CAD build for the part. Positions are in the model's coordinates, mm. A direction names the side the tool comes from. Round coordinates to 2 decimals unless told otherwise and drop trailing zeros. Loops run counter-clockwise (first coordinate to the right, second up) from the corner with the lowest first, then second, coordinate; pieces in that order, holes last.
```python
from build123d import *

# Parameters (mm, degrees)
F0_W     = 310.82517
F0_H     = 231.34768
F1_DEPTH = 189
F2_R     = 20
F3_R     = 13.644912
F3_R_2   = 26.127936
F3_R_3   = 16.173919
F4_DEPTH = 189.001
F5_T     = -10
F6_R     = 32.715141
F7_DEPTH = 189.001


with BuildPart() as f1:
    # F0 (on Front) → F1 (new body)
    with BuildSketch(Plane.XZ):
        Rectangle(F0_W, F0_H)
    extrude(amount=F1_DEPTH)

    # F2
    f2_edges = [f1.edges().sort_by_distance(p)[0] for p in [
        (155.412585, -94.5, 115.67384),
        (-155.412585, -94.5, 115.67384),
        (0, 0, 115.67384),
        (0, -189, 115.67384),
    ]]
    fillet(f2_edges, radius=F2_R)

    # F3 (on face) → F4 (cut, through all)
    with BuildSketch(Plane.XZ.offset(189)):
        with Locations((-105.628975, -68.58331)):
            Circle(F3_R)
        with Locations((-9.658518, -9.867162)):
            Circle(F3_R_2)
        with Locations((92.311822, 54.978933)):
            Circle(F3_R_3)
    extrude(amount=-F4_DEPTH, mode=Mode.SUBTRACT)

    # F5
    f5_openings = [f1.faces().sort_by_distance(p)[0] for p in [
        (0, -94.5, -115.67384),
    ]]
    offset(amount=F5_T, openings=f5_openings)

    # F6 (on face) → F7 (cut, through all)
    with BuildSketch(Plane(origin=(0, 0, 0), x_dir=(-1, 0, 0), z_dir=(0, 1, 0))):
        with Locations((-73.95748, -58.360144)):
            Circle(F6_R)
    extrude(amount=-F7_DEPTH, mode=Mode.SUBTRACT)


solid = f1.part
```
Item 1: 3-axis set-ups, long thin cutter, end or side, ignore diameter. For faces 4 (the cylindrical face through (2.036, -175.993, 102.822)), 5 (the cylindrical face through (-149.71, -95.82, 109.66)), 6 (the cylindrical face through (142.56, -95.68, 102.67)): which of +Z, -Z, +X, -X, +Y, -Y reach the whole face in a straight line?
Answers follow:
face 4: none
face 5: +Z, -X, +Y, -Y
face 6: -Z
Item 2: Flat gauge pins, fed straight in: P1, Ø1.5, axis at x = 123, y = -47.5, coming from the -Z side; P2, Ø19.5, axis at x = 92.31, z = 54.98, coming from the -Y side; P3, Ø1, axis at x = -20.5, y = -82, coming from the -Z side. Where does each tip first touch, or does it go through?
Answers follow:
P1: stops at z = 105.67
P2: passes through
P3: stops at z = -44.48
Item 3: Probe line 1 (X direction, y = -63, z = -105); line 2 (Y direction, x = -39, z = 16); line 3 (X direction, y = -127, z = 57). List the from-to ranges inside material, lowest first.
Answers follow:
line 1: x = -155.41 to -145.41, 145.41 to 155.41
line 2: y = -189 to -179, -10 to 0
line 3: x = -155.41 to -145.41, 66.22 to 76.26, 108.36 to 118.41, 145.41 to 155.41
Item 4: Cut at B-B, the plane x = 70. Give the cut face in (y, z).
Answers follow:
outline: (-189, -115.67) - (-179, -115.67) - (-179, -90.84) - (-189, -90.84) - close; (-189, -25.89) - (-179, -25.89) - (-179, 41.29) - (-10, 41.29) - (-10, -25.89) - (0, -25.89) - (0, 95.67) arc R20 ccw to (-20, 115.67) - (-169, 115.67) arc R20 ccw to (-189, 95.67) - close; (-10, -115.67) - (0, -115.67) - (0, -90.84) - (-10, -90.84) - close; hole (-179, 68.66) - (-10, 68.66) - (-10, 95.67) arc R10 ccw to (-20, 105.67) - (-169, 105.67) arc R10 ccw to (-179, 95.67) - close
Item 5: Two-plate mould, pull along X, no slides. Class faces 1 (the flat face through (-2, -93, 115.674)), 2 (the flat face through (155.413, -93, -11)), 3 (the cylindrical face through (81.049, -183.93, -90.297)): released by +X, released by -X, zero draft, split by the parting line, or undercut.
Answers follow:
face 1: zero draft
face 2: released by +X
face 3: undercut
Item 6: Cut at D-D, the plane z = 65.5. Give the cut face in (x, y).
Answers follow:
outline: (-155.41, -189) - (80.03, -189) - (80.03, 0) - (-155.41, 0) - close; (104.6, -189) - (155.41, -189) - (155.41, 0) - (104.6, 0) - close; hole (-145.41, -179) - (68.35, -179) - (68.35, -10) - (-145.41, -10) - close; hole (116.28, -179) - (145.41, -179) - (145.41, -10) - (116.28, -10) - close
Item 7: Cut at C-C, the plane y = -14.5. Give the cut face in (x, z).
Answers follow:
outline: (-155.41, -115.67) - (-145.41, -115.67) - (-145.41, 95.67) arc R10 cw to (-140.91, 104.03) - (140.91, 104.03) arc R10 cw to (145.41, 95.67) - (145.41, -115.67) - (155.41, -115.67) - (155.41, 95.67) arc R20 ccw to (140.91, 114.9) - (-140.91, 114.9) arc R20 ccw to (-155.41, 95.67) - close; circle Ø47.29 at (-105.63, -68.58); circle Ø72.26 at (-9.66, -9.87); circle Ø52.35 at (92.31, 54.98); hole circle Ø27.29 at (-105.63, -68.58); hole circle Ø52.26 at (-9.66, -9.87); hole circle Ø32.35 at (92.31, 54.98)
Item 8: Cut at A-A, the plane z = -77. Give the cut face in (x, y).
Answers follow:
outline: (-155.41, -189) - (-116.37, -189) - (-116.37, 0) - (-155.41, 0) - close; (-94.89, -189) - (47.07, -189) - (47.07, -179) - (-83.53, -179) - (-83.53, -10) - (47.07, -10) - (47.07, 0) - (-94.89, 0) - close; (100.84, -189) - (155.41, -189) - (155.41, 0) - (100.84, 0) - (100.84, -10) - (145.41, -10) - (145.41, -179) - (100.84, -179) - close; hole (-145.41, -179) - (-127.73, -179) - (-127.73, -10) - (-145.41, -10) - close
